Drawing for the job (mm, zero at the part's lowest x, y, z). A direction names the side the tool comes from. Give positions to 0.01 mm unless a question says otherwise; leave off trailing zeros. Loops run counter-clockwise (first coordinate to the right, second up) from the corner with the lowest first, then second, coordinate; pieces in that order, holes last. Notation, with made-up numbers: (-1.5, 3.25) -> (31.5, 3.25) arc R27 cw to (31.5, 32.25) -> close; hole circle Ø7 at (14.5, -31). An arc over 180 degrees is marked (long way). Write item = value, one per line.
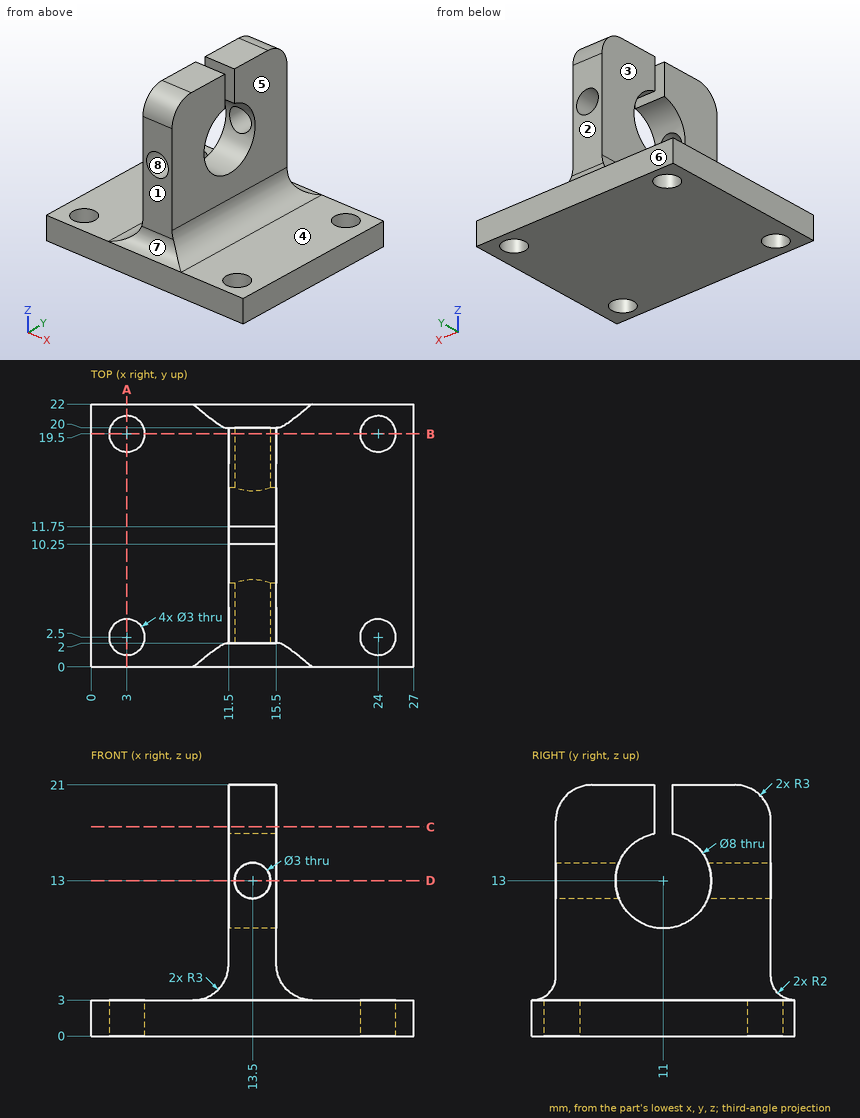
1) Slice it at A-A, the plane x = 3. List the corners of the cut face in (y, z).
Resolved:
outline = (0, 0) -> (1, 0) -> (1, 3) -> (0, 3) -> close; (4, 0) -> (18, 0) -> (18, 3) -> (4, 3) -> close; (21, 0) -> (22, 0) -> (22, 3) -> (21, 3) -> close
2) Slice it at C-C, the plane z = 17.5. List the corners of the cut face in (x, y), and give its area (3 significant figures).
Resolved:
outline = (11.5, 2) -> (15.5, 2) -> (15.5, 10.25) -> (11.5, 10.25) -> close; (11.5, 11.75) -> (15.5, 11.75) -> (15.5, 20) -> (11.5, 20) -> close
area = 66.0 mm²
3) Slice it at D-D, the plane z = 13. List the corners of the cut face in (x, y).
Resolved:
outline = (11.5, 2) -> (12, 2) -> (12, 7) -> (11.5, 7) -> close; (11.5, 15) -> (12, 15) -> (12, 20) -> (11.5, 20) -> close; (15, 2) -> (15.5, 2) -> (15.5, 7) -> (15, 7) -> close; (15, 15) -> (15.5, 15) -> (15.5, 20) -> (15, 20) -> close
4) Slice it at B-B, the plane y = 19.5. List the corners of the cut face in (x, z).
Resolved:
outline = (0, 0) -> (1.5, 0) -> (1.5, 3) -> (0, 3) -> close; (4.5, 0) -> (22.5, 0) -> (22.5, 3) -> (18.5, 3) arc R3 cw to (15.5, 6) -> (15.5, 19.66) -> (11.5, 19.66) -> (11.5, 6) arc R3 cw to (8.5, 3) -> (4.5, 3) -> close; (25.5, 0) -> (27, 0) -> (27, 3) -> (25.5, 3) -> close; hole circle Ø3 at (13.5, 13)
5) Pull direction Z, two halves, no side cores. Call the marked faces 6, 7 and 8: pulls with the +Z half, pulls with the -Z half, needs draft (parallel to the pull), parting line crosses it, or undercut.
Resolved:
face_6 = needs draft
face_7 = pulls with the +Z half
face_8 = undercut
6) Drill centre lines: line 1 along Y through (x, z) = (13, 7.75); line 2 along Z through (x, y) = (23.5, 7); line 3 along Y through (x, z) = (12.5, 14.25). Where is each one in solid material? Low to high. Write a range as [from, to].
Resolved:
line_1 = [2, 20]
line_2 = [0, 3]
line_3 = [2, 7.2], [14.8, 20]
7) Drop flat-ended pins along their axis: P1, Ø5, axis at x = 13.5, z = 11.5, coming from the -Y side; P2, Ø4.5, axis at x = 12.5, z = 19, coming from the +Y side; P3, Ø6.5, axis at y = 11, z = 13, coming from the -X side; P4, Ø12, axis at y = 12, z = 11, coming from the +X side. Give the stop position or say it passes through.
Resolved:
P1 = 2
P2 = 20
P3 = through
P4 = 15.67
8) Which spindle directions (+Z, -Z, +X, -X, +Y, -Y) get a long thin tool onto all of the face, cutting with end or side? Do the marked faces 1, 2, 3, 4 and 5. Say none if no direction does.
Resolved:
face_1 = +Z, +X, -X, -Y
face_2 = +Z, +X, -X, +Y
face_3 = +Z, -X, +Y, -Y
face_4 = +Z, +X, +Y, -Y
face_5 = +Z, +X, +Y, -Y
